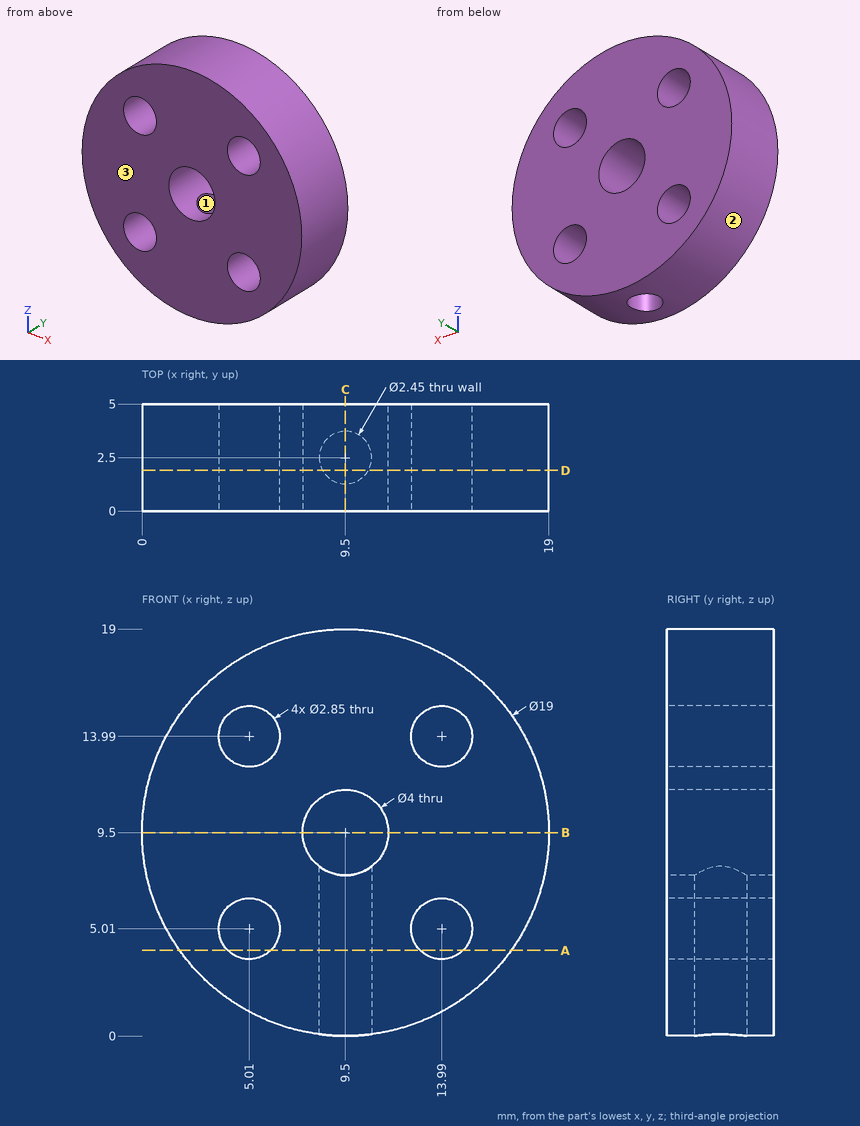
Could you check a few things on this drawing? It's one solid part, dimensions in mm from its lowest x, y, z. Give positions to 0.01 mm unless a question says otherwise; leave off trailing zeros. Write each loop counter-clockwise with the first axis right and the second up, starting at its lowest first coordinate (ties: lowest second). Pieces come first, ordered by that corner, then holes. Notation, with made-up numbers: (35, 59) -> (92, 59) arc R19 cw to (92, 87) -> close; hole circle Ø6 at (21, -39.75). An arc over 180 degrees is marked (long way). Write item = value, one per line.
(1) I'm going to push flat-ended pins straight in: P1, Ø1.5, axis at x = 11.5, y = 1, coming from the -Z side; P2, Ø3, axis at y = 4, z = 12.5, coming from the -X side. Where does each tip first touch, or does it pass through?
Worked out:
P1 = 0.08
P2 = 0.12
(2) Suppose I cut it at A-A on z = 4. Count the separate pieces of the cut face and the enclosed holes in it.
Worked out:
separate_pieces = 3
enclosed_holes = 1
(3) Suppose I cut it at D-D on y = 1.9. Write out the boundary of the cut face in (x, z) (3 decimals), then the cut area to 3 significant figures.
Worked out:
outline = (8.432, 0.06) -> (8.432, 7.809) arc R2 cw (long way) to (10.568, 7.809) -> (10.568, 0.06) arc R9.5 ccw (long way) to start; hole circle Ø2.85 at (5.01, 5.01); hole circle Ø2.85 at (5.01, 13.99); hole circle Ø2.85 at (13.99, 5.01); hole circle Ø2.85 at (13.99, 13.99)
area = 229 mm^2
(4) Suppose I cut it at C-C on x = 9.5. Write out the boundary of the cut face in (y, z) (3 decimals), then the cut area to 3 significant figures.
Worked out:
outline = (0, 0) -> (1.275, 0) -> (1.275, 7.5) -> (0, 7.5) -> close; (0, 11.5) -> (5, 11.5) -> (5, 19) -> (0, 19) -> close; (3.725, 0) -> (5, 0) -> (5, 7.5) -> (3.725, 7.5) -> close
area = 56.6 mm^2
(5) Suppose I cut it at B-B on z = 9.5. Write out the boundary of the cut face in (x, y).
Worked out:
outline = (0, 0) -> (7.5, 0) -> (7.5, 5) -> (0, 5) -> close; (11.5, 0) -> (19, 0) -> (19, 5) -> (11.5, 5) -> close
(6) I need wall thicknesses on probe 1 along Y at (x, z) = (9.5, 1.5) (3 decimals); probe 2 along Z at (x, y) = (13.75, 3.2) (1 decimal); probe 3 along X at (y, z) = (4.7, 13.25). Which ranges of each line are inside material? Lowest first, please. Write a range as from..to.
Worked out:
probe_1 = 0..1.275, 3.725..5
probe_2 = 1..3.6, 6.4..12.6, 15.4..18
probe_3 = 0.77..3.79, 6.23..12.77, 15.21..18.23
(7) Thinking about a two-plate mould opening in X: for the marked faces 1, 2 and 3, which applies, released by +X, released by -X, zero draft, split by the parting line, or undercut?
Worked out:
face_1 = undercut
face_2 = split by the parting line
face_3 = zero draft
